Geometry check sheet. Reference: the model listing, model coordinates, mm. A direction names the side the tool comes from. Round coordinates to 2 decimals unless told otherwise and drop trailing zeros. Order: outer loops, then holes, each group sorted by start corner. A loop starts at its lowest first (then second) coordinate and runs counter-clockwise, first axis right, second up. Notation, with made-up numbers: (-16.5, 27.5) -> (-10.5, 27.5) arc R17 ccw to (-10.5, 52.5) -> close; hole circle Ø6 at (26.25, 39). An arc over 180 degrees is marked (long way). Answer as a JSON object with one key per item and string values. Group by question number.
from build123d import *

# Parameters (mm, degrees)
SKETCH3_W           = 35
SKETCH3_H           = 30
SKETCH3_W_2         = 30
SKETCH3_H_2         = 35
BOSS_EXTRUDE3_DEPTH = 4
SKETCH4_W           = 30
SKETCH4_H           = 5
BOSS_EXTRUDE4_DEPTH = 50


with BuildPart() as part:
    # Sketch3 → Boss-Extrude3 (new body)
    with BuildSketch(Plane(origin=(0, 0, 0), x_dir=(1, 0, 0), z_dir=(0, 1, 0))):
        with Locations((-32.5, 0)):
            Rectangle(SKETCH3_W, SKETCH3_H)
        Rectangle(SKETCH3_W_2, SKETCH3_H)
        with Locations((0, -32.5)):
            Rectangle(SKETCH3_W_2, SKETCH3_H_2)
        with Locations((32.5, 0)):
            Rectangle(SKETCH3_W, SKETCH3_H)
        with Locations((0, 32.5)):
            Rectangle(SKETCH3_W_2, SKETCH3_H_2)
    extrude(amount=BOSS_EXTRUDE3_DEPTH)

    # Sketch4 → Boss-Extrude4 (add)
    with BuildSketch(Plane(origin=(0, 4, 0), x_dir=(1, 0, 0), z_dir=(0, 1, 0))):
        with Locations((0, -47.5)):
            Rectangle(SKETCH4_W, SKETCH4_H)
        with Locations((0, 47.5)):
            Rectangle(SKETCH4_W, SKETCH4_H)
    extrude(amount=BOSS_EXTRUDE4_DEPTH)


solid = part.part
Item 1: Depth check by flat-ended pin: pin 1 Ø1.2 at (x, y) = (-24.5, 2) entering from +Z; pin 2 Ø17.5 at (y, z) = (17.5, 41) entering from +X; pin 3 Ø3 at (x, y) = (36, 3) entering from -Z. Enter the tip coordinate at first touch or a pass-through.
Item 2: Mould release check, pull along Z, two halves, no side actions. Record for faces 6 (the flat face through (0, 27, -50)), 7 (the flat face through (-1, 4, -1)), 8 (the flat face through (-50, 2, 0)), 9 (the flat face through (0, 29, 45)): pulls with the +Z half, pulls with the -Z half, needs draft (parallel to the pull), parting line crosses it, or undercut.
Item 3: Set-up check for faces 1 (the flat face through (-15, 21, 46)), 2 (the flat face through (0, 29, -45)), 3 (the flat face through (15, 18.9, -45.4)), 4 (the flat face through (-15, 18.9, -45.4)), 5 (the flat face through (32, 2, 15)): record each of +Z, -Z, +X, -X, +Y, -Y from which the full face is reachable in a straight line by a thin tool's end or side.
Item 4: Thickness scan on L1, parallel to Z at x = 8, y = 21; L2, parallel to Y at x = 12, z = -2.5; L3, parallel to X at y = 12.5, z = 45.5. Record the ranges inside material, lowest first.
Item 5: Sectioned sample at A-A, the plane y = 14. Enter the section's corners in (x, z).
Item 6: Sectioned sample at B-B, the plane x = -2. Enter the section's corners in (y, z).
Item 7: Sectioned sample at C-C, the plane z = 41. Enter the section's corners in (x, y), then the cut area to 3 significant figures.
Item 8: Sectioned sample at D-D, the plane x = -38.5. Enter the section's corners in (y, z).
Result:
{
 "1": {"pin 1": "stops at z = 15", "pin 2": "stops at x = 15", "pin 3": "stops at z = -15"},
 "2": {"face 6": "pulls with the -Z half", "face 7": "undercut", "face 8": "needs draft", "face 9": "undercut"},
 "3": {"face 1": "+Z, -X, +Y, -Y", "face 2": "+X, -X, +Y", "face 3": "-Z, +X, +Y, -Y", "face 4": "-Z, -X, +Y, -Y", "face 5": "+Z, +X, +Y, -Y"},
 "4": {"L1": "z = -50 to -45, 45 to 50", "L2": "y = 0 to 4", "L3": "x = -15 to 15"},
 "5": {"outline": "(-15, -50) -> (15, -50) -> (15, -45) -> (-15, -45) -> close; (-15, 45) -> (15, 45) -> (15, 50) -> (-15, 50) -> close"},
 "6": {"outline": "(0, -50) -> (54, -50) -> (54, -45) -> (4, -45) -> (4, 45) -> (54, 45) -> (54, 50) -> (0, 50) -> close"},
 "7": {"outline": "(-15, 0) -> (15, 0) -> (15, 4) -> (-15, 4) -> close", "area": "120 mm2"},
 "8": {"outline": "(0, -15) -> (4, -15) -> (4, 15) -> (0, 15) -> close"}
}
